Part model, mm, in its own coordinate system. A direction names the side the tool comes from. Round coordinates to 2 decimals unless told otherwise and drop trailing zeros. Loops run counter-clockwise (first coordinate to the right, second up) from the corner with the lowest first, then second, coordinate; pieces in that order, holes last.
from build123d import *

# Parameters (mm, degrees)
CHAMFER_1_SIZE           = 1
CUT_EXTRUDE_1_DEPTH      = 49.093658626
CUT_EXTRUDE_1_DEPTH_BACK = 49.093658626
SKETCH_2_R               = 1


with BuildPart() as part:
    # 草圖1 → 旋轉1 (revolve)
    with BuildSketch(Plane(origin=(0, 0, 0), x_dir=(0, 0, -1), z_dir=(1, 0, 0)), mode=Mode.PRIVATE) as revolve_1_sk:
        Polygon((0, 0), (0, 12), (10, 12), (10, 6), (45, 6), (45, 0), align=None)
    revolve(revolve_1_sk.sketch.rotate(Axis((0, 0, 0), (0, 0, -1)), 90), axis=Axis((0, 0, 0), (0, 0, -1)))

    # 導角1
    chamfer_1_edges = [part.edges().sort_by_distance(p)[0] for p in [
        (-6, 0, -45),
        (-12, 0, 0),
    ]]
    chamfer(chamfer_1_edges, length=CHAMFER_1_SIZE)

    # 草圖2 → 伸長1 (cut, two sides: drawn at the far end of the back side and taken through both)
    with BuildSketch(Plane(origin=(0, 0, 0), x_dir=(0, 0, -1), z_dir=(1, 0, 0)).offset(-CUT_EXTRUDE_1_DEPTH_BACK)):
        with Locations((41, 0)):
            Circle(SKETCH_2_R)
    extrude(amount=CUT_EXTRUDE_1_DEPTH + CUT_EXTRUDE_1_DEPTH_BACK, mode=Mode.SUBTRACT)


solid = part.part
1) Slice it at D-D, the plane z = -31.5. Give the cut face in (x, y).
Values:
outline: circle Ø12 at (0, 0)
2) Slice it at C-C, the plane z = -41. Give the cut face in (x, y).
Values:
outline: (-5.92, -1) arc R6 ccw to (5.92, -1) - close; (-5.92, 1) - (5.92, 1) arc R6 ccw to start
3) Slice it at A-A, the plane y = 0. Give the cut face in (x, z).
Values:
outline: (-12, -10) - (-6, -10) - (-6, -40) - (6, -40) - (6, -10) - (12, -10) - (12, -1) - (11, 0) - (-11, 0) - (-12, -1) - close; (-6, -44) - (-5, -45) - (5, -45) - (6, -44) - (6, -42) - (-6, -42) - close
4) Drop flat-ended pins along their axis: pin 1 Ø5 at (x, z) = (9, -20.5) entering from -Y; pin 2 Ø1 at (x, y) = (2, -9) entering from -Z; pin 3 Ø5 at (x, z) = (2.5, -12) entering from -Y; pin 4 Ø10 at (y, z) = (-5.5, -6.5) entering from +X. Give the stop position or say it passes through.
Values:
pin 1: passes through
pin 2: stops at z = -10
pin 3: stops at y = -11.96
pin 4: stops at x = 11.99
5) Mould opens along Y. For faces 3 (the face through (0, 0, -42)), 4 (the face through (0, 0, -45)), 5 (the face through (11.446, -3.604, -5.563)) say: released by +Y, released by -Y, zero draft, split by the parting line, or undercut.
Values:
face 3: undercut
face 4: zero draft
face 5: split by the parting line
6) Slice it at B-B, the plane x = 0. Give the cut face in (y, z).
Values:
outline: (-12, -10) - (-6, -10) - (-6, -44) - (-5, -45) - (5, -45) - (6, -44) - (6, -10) - (12, -10) - (12, -1) - (11, 0) - (-11, 0) - (-12, -1) - close; hole circle Ø2 at (0, -41)
7) Tool access for faces 1 (the face through (0, 0, 0)), 2 (the face through (5.723, -1.802, -27.238)): list every direction of +Z, -Z, +X, -X, +Y, -Y with a clear straight run to the whole face (end or side of a thin tool).
Values:
face 1: +Z, +X, -X, +Y, -Y
face 2: -Z
8) Wall check: line 1 along Z through (x, y) = (-2.5, 0); line 2 along Y through (x, z) = (-0.25, -41); line 3 along Z through (x, y) = (2.5, -7). Give the ranges that are in metal, low to high.
Values:
line 1: z = -45 to -42, -40 to 0
line 2: y = -5.99 to -1, 1 to 5.99
line 3: z = -10 to 0
